Part model, mm, in its own coordinate system. A direction names the side the tool comes from. Coordinates: 2 decimals unless noted, no trailing zeros. Order: outer loops, then holes, each group sorted by start corner. A loop starts at its lowest first (then second) coordinate and runs counter-clockwise, first axis right, second up.
1) Cut at A-A (z = 22). List the corners of the cut face in (x, y).
2) Tool access for faces 1 (the flat face through (30, 20, 30)), 2 (the flat face through (24, 20, 0)): list every direction of +Z, -Z, +X, -X, +Y, -Y with a clear straight run to the whole face (end or side of a thin tool).
3) Pin check, flat tips, straight feed: pin 1 Ø5 at (x, y) = (16, 14.5) entering from +Z; pin 2 Ø3 at (x, y) = (18.5, 6) entering from +Z; pin 3 Ø1.5 at (x, z) = (14, 7.5) entering from +Y; pin 4 Ø12 at (x, y) = (5.5, 29) entering from +Z. Stop position of each tip, or through.
4) Cut at C-C (x = 24). List the corners of the cut face in (y, z).
5) Cut at B-B (y = 10). List the corners of the cut face in (x, z).
6) Cut at D-D (z = 32.5). List the corners of the cut face in (x, y).
7) Wall check: L1, parallel to X at y = 33.5, z = 31; L2, parallel to Y at x = 25, z = 28.5; L3, parallel to Y at x = 38.5, z = 33. Give the ranges that are in metal, low to high.
```python
from build123d import *

# Parameters (mm, degrees)
SKETCH1_W           = 40
SKETCH1_H           = 40
BOSS_EXTRUDE1_DEPTH = 40
CUT_EXTRUDE1_DEPTH  = 40
CUT_EXTRUDE3_DEPTH  = 20
CUT_EXTRUDE4_DEPTH  = 20


with BuildPart() as part:
    # Sketch1 → Boss-Extrude1 (new body)
    with BuildSketch(Plane.XY):
        with Locations((20, 20)):
            Rectangle(SKETCH1_W, SKETCH1_H)
    extrude(amount=BOSS_EXTRUDE1_DEPTH)

    # Sketch2 → Cut-Extrude1 (cut)
    with BuildSketch(Plane.XY.offset(40)):
        Polygon((0, 0), (20, 40), (0, 40), align=None)
    extrude(amount=-CUT_EXTRUDE1_DEPTH, mode=Mode.SUBTRACT)

    # Sketch3 → Cut-Extrude3 (cut)
    with BuildSketch(Plane(origin=(40, 0, 0), x_dir=(0, 0, -1), z_dir=(1, 0, 0))):
        Polygon((-20, 0), (-40, 40), (-40, 0), align=None)
    extrude(amount=-CUT_EXTRUDE3_DEPTH, mode=Mode.SUBTRACT)

    # Sketch5 → Cut-Extrude4 (cut)
    with BuildSketch(Plane(origin=(17.777777778, -8.888888889, 17.777777778), x_dir=(0.745355992, 0.298142397, -0.596284794), z_dir=(0.666666667, -0.333333333, 0.666666667))):
        Polygon((2.98142397, 53.66563146), (2.98142397, 8.94427191), (-23.85139176, 17.88854382), align=None)
    extrude(amount=CUT_EXTRUDE4_DEPTH, mode=Mode.SUBTRACT)


solid = part.part
```
Geometry check:
1. outline: (0, 0) - (18, 0) - (20, 4) - (40, 4) - (40, 40) - (20, 40) - close
2. face 1: +Z, +X, -Y
2. face 2: -Z, +X, -X, +Y, -Y
3. pin 1: stops at z = 34.05
3. pin 2: stops at z = 26.18
3. pin 3: stops at y = 29.5
3. pin 4: passes through
4. outline: (0, 0) - (40, 0) - (40, 40) - (0, 20) - close
5. outline: (5, 0) - (40, 0) - (40, 25) - (20, 25) - (5, 40) - close
6. outline: (0, 0) - (7.5, 0) - (20, 25) - (40, 25) - (40, 40) - (20, 40) - close
7. L1: x = 16.75 to 40
7. L2: y = 17 to 40
7. L3: y = 26 to 40
